```python
from build123d import *
from build123d.topology import SkipClean

# Parameters (mm, degrees)
BOSS_EXTRU_1_START      = 3.5
ESQUISSE1_R             = 2
BOSS_EXTRU_1_DEPTH      = 3
BOSS_EXTRU_2_START      = 6.5
BOSS_EXTRU_2_DEPTH      = 3.3
BOSS_EXTRU_5_START      = 7.3
ESQUISSE1_12_R          = 2
BOSS_EXTRU_5_DEPTH      = 2.5
BOSS_EXTRU_3_DEPTH      = 6.5
BOSS_EXTRU_4_START      = 0.5
BOSS_EXTRU_4_DEPTH      = 6
CONG_4_R                = 12
FILLET1_R               = 0.5
FILLET2_R               = 1
CHAMFER1_SIZE           = 2
ENL_V_START             = 3.5
ESQUISSE2_W             = 8
ESQUISSE2_H             = 18
ENL_V_MAT_EXTRU_1_DEPTH = 1
ENL_V_MAT_EXTRU_3_REACH = 52
ESQUISSE4_R             = 0.75
ESQUISSE5_W             = 21.366750419
ESQUISSE5_H             = 3.6
ENL_V_MAT_EXTRU_4_DEPTH = 1.1
CONG_5_R                = 1.1
ENL_V_MAT_EXTRU_5_REACH = 54.192
ESQUISSE12_R            = 0.75


# Some blends are built 0.0001 mm under size
with BuildPart() as part:
    # Esquisse1 → Boss.-Extru.1 (new body)
    with BuildSketch(Plane(origin=(0, 0, 0), x_dir=(0, 0, -1), z_dir=(1, 0, 0)).offset(BOSS_EXTRU_1_START)):
        with BuildLine():
            Line((30, 10), (0, 10))
            Line((0, 10), (0, 8))
            ThreePointArc((0, 8), (-8, 0), (0, -8))
            Line((0, -8), (30.291756081, -8))
            Line((30.291756081, -8), (30.291756081, 0))
            ThreePointArc((30.291756081, 0), (30.728647581, 2.879587526), (32, 5.5))
            Line((32, 5.5), (32, 8))
            Line((32, 8), (30, 10))
        make_face()
        Circle(ESQUISSE1_R, mode=Mode.SUBTRACT)
    extrude(amount=BOSS_EXTRU_1_DEPTH)

    # Esquisse1<8> → Boss.-Extru.2 (add)
    with BuildSketch(Plane(origin=(0, 0, 0), x_dir=(0, 0, -1), z_dir=(1, 0, 0)).offset(BOSS_EXTRU_2_START)):
        with BuildLine():
            Line((30, 10), (9.5, 10))
            Line((9.5, 10), (9.5, -8))
            Line((9.5, -8), (30.291756081, -8))
            Line((30.291756081, -8), (30.291756081, 0))
            ThreePointArc((30.291756081, 0), (30.728647581, 2.879587526), (32, 5.5))
            Line((32, 5.5), (32, 8))
            Line((32, 8), (30, 10))
        make_face()
    extrude(amount=BOSS_EXTRU_2_DEPTH)

    # Esquisse1<12> → Boss.-Extru.5 (add)
    with BuildSketch(Plane(origin=(0, 0, 0), x_dir=(0, 0, -1), z_dir=(1, 0, 0)).offset(BOSS_EXTRU_5_START)):
        with BuildLine():
            Line((40, 8), (32, 8))
            Line((32, 8), (32, 7))
            Line((32, 7), (32, 5.5))
            ThreePointArc((32, 5.5), (30.728647581, 2.879587526), (30.291756081, 0))
            Line((30.291756081, 0), (30.291756081, -8))
            Line((30.291756081, -8), (40, -8))
            ThreePointArc((40, -8), (48, 0), (40, 8))
        make_face()
        with Locations((40, 0)):
            Circle(ESQUISSE1_12_R, mode=Mode.SUBTRACT)
    extrude(amount=BOSS_EXTRU_5_DEPTH)

    # Esquisse1<9> → Boss.-Extru.3 (add)
    with BuildSketch(Plane(origin=(0, 0, 0), x_dir=(0, 0, -1), z_dir=(1, 0, 0))):
        with BuildLine():
            Line((0, 10), (2, 8))
            Line((2, 8), (28, 8))
            ThreePointArc((28, 8), (29.530733729, 8.30448187), (30.828427125, 9.171572875))
            Line((30.828427125, 9.171572875), (30, 10))
            Line((30, 10), (0, 10))
        make_face()
        with BuildLine():
            Line((0, 5.5), (28.791756081, 5.5))
            Line((28.791756081, 5.5), (28.791756081, -8))
            Line((28.791756081, -8), (30.291756081, -8))
            Line((30.291756081, -8), (30.291756081, 0))
            ThreePointArc((30.291756081, 0), (30.728647581, 2.879587526), (32, 5.5))
            Line((32, 5.5), (32, 7))
            Line((32, 7), (0, 7))
            ThreePointArc((0, 7), (-6.467156728, 2.678784027), (-4.949747468, -4.949747468))
            Line((-4.949747468, -4.949747468), (-3.889087297, -3.889087297))
            ThreePointArc((-3.889087297, -3.889087297), (-5.081337429, 2.104758878), (0, 5.5))
        make_face()
    extrude(amount=BOSS_EXTRU_3_DEPTH)

    # Esquisse1<10> → Boss.-Extru.4 (add)
    with BuildSketch(Plane(origin=(0, 0, 0), x_dir=(0, 0, -1), z_dir=(1, 0, 0)).offset(BOSS_EXTRU_4_START)):
        with BuildLine():
            Line((2, 8), (0, 10))
            Line((0, 10), (0, 8))
            ThreePointArc((0, 8), (-7.39103626, 3.061467459), (-5.656854249, -5.656854249))
            Line((-5.656854249, -5.656854249), (-4.949747468, -4.949747468))
            ThreePointArc((-4.949747468, -4.949747468), (-6.467156728, 2.678784027), (0, 7))
            Line((0, 7), (32, 7))
            Line((32, 7), (32, 8))
            Line((32, 8), (30.828427125, 9.171572875))
            ThreePointArc((30.828427125, 9.171572875), (29.530733729, 8.30448187), (28, 8))
            Line((28, 8), (2, 8))
        make_face()
    extrude(amount=BOSS_EXTRU_4_DEPTH)

    # Congé4
    # the kernel refuses this fillet: 12 mm, written as the material it takes off along each edge
    with BuildSketch(Plane(origin=(-11.583123952, 8, -2), x_dir=(0, 0, -1), z_dir=(1, 0, 0))) as cong_4_piece_1:
        with BuildLine():
            CenterArc((4.633249581, 12), CONG_4_R, 236.442690238, 33.557309762)
            Line((-2, 2), (-2.132664992, 1.8))
            ThreePointArc((-2.132664992, 1.8), (-1.169705627, 0.830294373), (-0.169705627, -0.169705627))
            Line((-0.169705627, -0.169705627), (0, -0.24))
            Line((0, -0.24), (4.633249581, -0.24))
            Line((4.633249581, -0.24), (4.633249581, 0))
        make_face()
    extrude(amount=12.083123952, mode=Mode.SUBTRACT)

    # Fillet1
    # the kernel refuses this fillet: 0.5 mm, written as the material it adds along each edge
    with BuildSketch(Plane(origin=(0.5, 20, -6.633249581), x_dir=(0, -0.7713363788823462, 0.6364276790120538), z_dir=(0, 0.6364276790120538, 0.7713363788823462))) as fillet1_piece_1_section:
        with BuildLine():
            CenterArc((12 + FILLET1_R, -FILLET1_R), FILLET1_R, 90, 90)
            Line((12 + FILLET1_R, 0), (12, 0))
            Line((12, 0), (12, -FILLET1_R))
        make_face()
    fillet1_piece_1 = revolve(axis=Axis((0.5, 20, -6.633249581), (1, 0, 0)), revolution_arc=39.525953359, mode=Mode.PRIVATE)
    fillet1_piece_1 = split(fillet1_piece_1, bisect_by=Plane(origin=(0.358961784, 10, -3.12843374), z_dir=(0, -1, 0)), keep=Keep.TOP, mode=Mode.PRIVATE)
    fillet1_piece_1 = split(fillet1_piece_1, bisect_by=Plane(origin=(0.358961784, 8.375840896, 0), z_dir=(0, 0, -1)), keep=Keep.TOP, mode=Mode.PRIVATE)
    add(fillet1_piece_1)
    with BuildSketch(Plane(origin=(0.5, 8, -28), x_dir=(-1, 0, 0), z_dir=(0, 0, 1))) as fillet1_piece_2:
        with BuildLine():
            CenterArc((FILLET1_R, FILLET1_R), FILLET1_R, 180, 90)
            Line((0, FILLET1_R), (0, 0))
            Line((0, 0), (FILLET1_R, 0))
        make_face()
    extrude(amount=21.366750419)
    with BuildSketch(Plane(origin=(0.5, 7, 0), x_dir=(-1, 0, 0), z_dir=(0, 0, -1))) as fillet1_piece_3:
        with BuildLine():
            CenterArc((FILLET1_R, FILLET1_R), FILLET1_R, 180, 90)
            Line((0, FILLET1_R), (0, 0))
            Line((0, 0), (FILLET1_R, 0))
        make_face()
    extrude(amount=32)
    with BuildSketch(Plane(origin=(0.5, 0, 0), x_dir=(0, -0.7071067811865441, 0.7071067811865509), z_dir=(0, -0.7071067811865509, -0.7071067811865441))) as fillet1_piece_4:
        with BuildLine():
            CenterArc((7 + FILLET1_R, FILLET1_R), FILLET1_R, 180, 90)
            Line((7 + FILLET1_R, 0), (7, 0))
            Line((7, 0), (7, FILLET1_R))
        make_face()
    revolve(axis=Axis((0.5, 0, 0), (-1, 0, 0)), revolution_arc=135)
    with BuildSketch(Plane(origin=(0.5, 12, -28), x_dir=(0, -0.7071067811865426, -0.7071067811865523), z_dir=(0, 0.7071067811865523, -0.7071067811865426))) as fillet1_piece_5:
        with BuildLine():
            CenterArc((4 + FILLET1_R, FILLET1_R), FILLET1_R, 180, 90)
            Line((4 + FILLET1_R, 0), (4, 0))
            Line((4, 0), (4, FILLET1_R))
        make_face()
    revolve(axis=Axis((0.5, 12, -28), (-1, 0, 0)), revolution_arc=45)

    # Fillet2
    fillet2_edges = [part.edges().sort_by_distance(p)[0] for p in [
        (3.5, 8, 0),
    ]]
    fillet(fillet2_edges, radius=FILLET2_R)

    # Chamfer1
    chamfer1_edges = [part.edges().sort_by_distance(p)[0] for p in [
        (9.8, 1, -9.5),
    ]]
    chamfer(chamfer1_edges, length=CHAMFER1_SIZE)

    # Symétrie1: part across plane


with BuildPart() as part_1:
    add(part.part)
    add(part.part.mirror(Plane(origin=(0, 0, 0), x_dir=(0, 0, 1), z_dir=(1, 0, 0))))

    # Esquisse2 → Enlèv. mat.-Extru.1 (cut)
    with SkipClean():  # the faces are left unmerged after this step: merging them gives an invalid solid
        with BuildSketch(Plane(origin=(0, 0, 0), x_dir=(0, 0, -1), z_dir=(1, 0, 0)).offset(ENL_V_START)):
            with Locations((-4, 1)):
                Rectangle(ESQUISSE2_W, ESQUISSE2_H)
        extrude(amount=-ENL_V_MAT_EXTRU_1_DEPTH, mode=Mode.SUBTRACT)

    # Esquisse4 → Enlèv. mat.-Extru.3 (cut, up to next)
    with BuildSketch(Plane.XY, mode=Mode.PRIVATE) as enl_v_mat_extru_3_sk1:
        with Locations((2.75, -3.8608)):
            Circle(ESQUISSE4_R)
    enl_v_mat_extru_3_tool1 = extrude(enl_v_mat_extru_3_sk1.sketch, amount=-ENL_V_MAT_EXTRU_3_REACH, mode=Mode.PRIVATE) & part_1.part
    add(enl_v_mat_extru_3_tool1.solids().sort_by_distance((2.75, -3.8608, 0))[0], mode=Mode.SUBTRACT)

    # Esquisse5 → Enlèv. mat.-Extru.4 (cut, symmetric)
    with SkipClean():  # the faces are left unmerged after this step: merging them gives an invalid solid
        with BuildSketch(Plane(origin=(0, 0, 0), x_dir=(0, 0, -1), z_dir=(1, 0, 0))):
            with Locations((17.316624791, 8.2)):
                Rectangle(ESQUISSE5_W, ESQUISSE5_H)
        extrude(amount=ENL_V_MAT_EXTRU_4_DEPTH, both=True, mode=Mode.SUBTRACT)

    # Congé5
    cong_5_edges = [part_1.edges().sort_by_distance(p)[0] for p in [
        (1.1, 6.4, -17.31662479),
        (-1.1, 6.4, -17.31662479),
    ]]
    fillet(cong_5_edges, radius=CONG_5_R - 0.0001)  # a hair under: the kernel refuses the full size

    # Esquisse10 → Enlèvement de matière-Révolution1 (revolve, cut)
    with BuildSketch(Plane.XY, mode=Mode.PRIVATE) as enl_vement_de_mati_re_r_volution1_sk:
        Polygon((-6.5, 5.15), (-5.9, 5.15), (-5.9, 4.5), (5.9, 4.5), (5.9, 5.15), (6.5, 5.15), (6.5, 2), (-6.5, 2), align=None)
    revolve(enl_vement_de_mati_re_r_volution1_sk.sketch.rotate(Axis((-6.5, 0, 0), (1, 0, 0)), 90), axis=Axis((-6.5, 0, 0), (1, 0, 0)), mode=Mode.SUBTRACT)

    # Esquisse12 → Enlèv. mat.-Extru.5 (cut, up to next)
    with BuildSketch(Plane(origin=(0, 10, 0), x_dir=(1, 0, 0), z_dir=(0, 1, 0)), mode=Mode.PRIVATE) as enl_v_mat_extru_5_sk1:
        with Locations(Location((-2.75, 4.322277882, 0), (0, 0, 270))):
            Circle(ESQUISSE12_R)
    enl_v_mat_extru_5_tool1 = extrude(enl_v_mat_extru_5_sk1.sketch, amount=-ENL_V_MAT_EXTRU_5_REACH, mode=Mode.PRIVATE) & part_1.part
    add(enl_v_mat_extru_5_tool1.solids().sort_by_distance((-2.75, 10, -4.322278))[0], mode=Mode.SUBTRACT)


solid = part_1.part
```
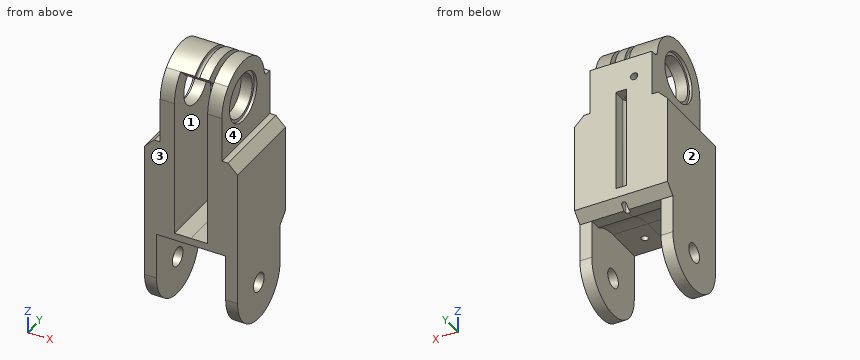
Check sheet for the modelled part. Datum: model origin and axes. Units: mm. Face numbers are marked on the shaded views. Give positions to 0.01 mm unless a question says otherwise; leave off trailing zeros. Write each loop counter-clockwise with the first axis right and the second up, starting at its lowest first coordinate (ties: lowest second). Pieces come first, ordered by that corner, then holes. Notation, with made-up numbers: (67, 8.25) -> (98, 8.25) arc R13 cw to (98, 28.25) -> close; hole circle Ø4 at (62.25, -38.75). An arc over 180 degrees is marked (long way). Use CSV: the item, a comma, the result in double quotes. Start each with the question number.
Q1. Cross-section at A-A on z = -36.5. Enter the section's corners in (x, y).
Q2. Scan lines: line 1 along X through (y, z) = (-6.75, -37.5); line 2 along X through (y, z) = (-4.75, -3); line 3 along Y through (x, z) = (-8.5, -40). Record each from-to range of solid material in increasing order.
Q3. Depth check by flat-ended pin: P1, Ø3, axis at x = -4, y = 7, coming from the -Z side; P2, Ø3, axis at x = -1.5, z = -18, coming from the -Y side; P3, Ø4, axis at x = 4.5, y = 3, coming from the -Z side; P4, Ø1, axis at x = 1, z = -25.5, coming from the +Y side. Enter the tip coordinate at first touch or a pass-through.
Q4. Cross-section at B-B on x = 4.5. Enter the section's corners in (y, z), and give its area (3 significant figures).
Q5. Cross-section at D-D on y = 1.25. Count the separate pieces of the cut face and the enclosed holes in it, and give its area (3 significant figures).
Q6. Release check for a two-part mould opening along X. For the marked faces 1, 2, 3 and 4 record: +X half, -X half, draft (parallel to the pull), parting line (faces both ways), or undercut.
Working result:
1,outline,"(-9.8, -8) -> (-7.3, -8) -> (-7.3, 8) -> (-9.8, 8) -> close; (7.3, -8) -> (9.8, -8) -> (9.8, 8) -> (7.3, 8) -> close"
2,line 1,"x = -9.8 to -7.3, 7.3 to 9.8"
2,line 2,"x = -6.5 to -3.5, 3.5 to 6.5"
2,line 3,"y = -8 to -2, 2 to 8"
3,P1,"stops at z = -32"
3,P2,"stops at y = 5.5"
3,P3,"stops at z = -31.68"
3,P4,"stops at y = 10"
4,outline,"(-8, -30.29) -> (0, -30.29) arc R9.71 cw to (5.5, -32) -> (8, -32) -> (10, -30) -> (10, 0) -> (8.94, 0) arc R1 cw to (7.95, 0.89) arc R8 ccw to (-8, 0) -> close; hole circle Ø9 at (0, 0)"
4,area,"591 mm^2"
5,separate pieces,"5"
5,enclosed holes,"0"
5,area,"407 mm^2"
6,face 1,"undercut"
6,face 2,"-X half"
6,face 3,"draft"
6,face 4,"+X half"
